Geometry check sheet. Reference: drawing and pictorial views, mm from the part's lowest x, y, z. Give positions to 0.01 mm unless a question says otherwise; leave off trailing zeros. Write each loop counter-clockwise with the first axis right and the second up, starting at its lowest first coordinate (ties: lowest second). Pieces come first, ordered by that corner, then holes. Notation, with made-up numbers: M 55,-17.75 L 107,-17.75 A10 cw 107,-8.75 Z; hole C -37.75,29.5 d7. An arc over 180 degrees is marked long. Write each question's results on one line, items separated by ' | '. Start each with the question number.
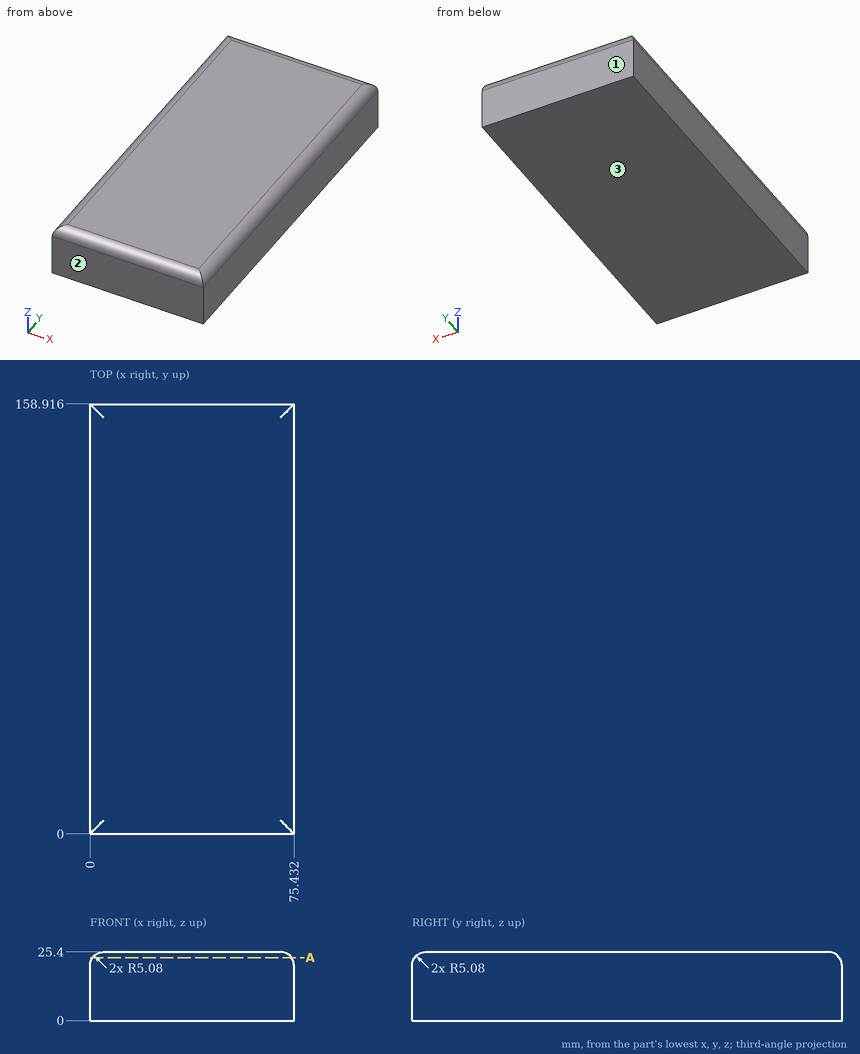
Q1. Scan lines: L1, parallel to Y at x = 7, z = 21.25 (1 decimal); L2, parallel to Y at x = 67, z = 22.75 (1 decimal); L3, parallel to X at y = 62, z = 22.5. Record each from-to range of solid material in increasing order.
Q2. Depth check by flat-ended pin: pin 1 Ø4 at (x, z) = (23, 22.5) entering from -Y. Enter the tip coordinate at first touch or a pass-through.
Q3. Release check for a two-part mould opening along Y. For the marked faces 1, 2 and 3 record: pulls with the +Y half, pulls with the -Y half, needs draft (parallel to the pull), parting line crosses it, or undercut.
Q4. Section check A-A on z = 23.25. Record the boundary of the cut face in (x, y) (1 decimal).
Check result:
1) L1: 0.1 to 158.8 | L2: 0.6 to 158.3 | L3: 0.49 to 74.94
2) pin 1: y = 0
3) face 1: pulls with the +Y half | face 2: pulls with the -Y half | face 3: needs draft
4) outline: M 0.9,0.9 L 74.5,0.9 L 74.5,158 L 0.9,158 Z
